Work out the finished part from the listing and answer in its coordinate system (mm). A direction names the side the tool comes from. Coordinates: 2 decimals unless noted, no trailing zeros. Write each loop counter-clockwise with the first axis right and the second up, starting at its lowest first coordinate (ties: lowest second). Pieces come first, ordered by that corner, then holes. Notation, with made-up numbers: M 75.5,80 L 87.5,80 A30 ccw 87.5,118 Z; hole C 44,7.25 d2. An arc over 180 degrees is marked long. Use CSV: the item, a comma, the result in double quotes.
Autodesk Inventor part; units mm, degrees
ref_plane "YZ Plane" through (0, 0, 0) normal (1, 0, 0) x (0, 1, 0)
ref_plane "XZ Plane" through (0, 0, 0) normal (0, 1, 0) x (-1, 0, 0)
ref_plane "XY Plane" through (0, 0, 0) normal (0, 0, 1) x (1, 0, 0)
sketch "Skizze1" plane through (0, 0, 0) normal (0, 0, 1) x (1, 0, 0)
  line L0 (-40.0777, 35.7212) -> (39.9223, 35.7212)
  line L1 (39.9223, 35.7212) -> (39.9223, -47.2788)
  line L2 (39.9223, -47.2788) -> (-40.0777, -47.2788)
  line L3 (-40.0777, -47.2788) -> (-40.0777, 35.7212)
  line L4 (-38.4777, 34.1212) -> (38.3223, 34.1212)
  line L5 (38.3223, 34.1212) -> (38.3223, -45.6788)
  line L6 (38.3223, -45.6788) -> (-38.4777, -45.6788)
  line L7 (-38.4777, -45.6788) -> (-38.4777, 34.1212)
  line L8 (-36.9777, 32.6212) -> (36.8223, 32.6212)
  line L9 (36.8223, 32.6212) -> (36.8223, -44.1788)
  line L10 (36.8223, -44.1788) -> (-36.9777, -44.1788)
  line L11 (-36.9777, -44.1788) -> (-36.9777, 32.6212)
  line L12 (-5.0777, -45.6788) -> (4.9223, -45.6788)
  line L13 (4.9223, -45.6788) -> (4.9223, -41.6788)
  line L14 (4.9223, -41.6788) -> (-5.0777, -41.6788)
  line L15 (-5.0777, -41.6788) -> (-5.0777, -45.6788)
  line L16 (-5.0777, 34.1212) -> (4.9223, 34.1212)
  line L17 (4.9223, 34.1212) -> (4.9223, 30.1212)
  line L18 (4.9223, 30.1212) -> (-5.0777, 30.1212)
  line L19 (-5.0777, 30.1212) -> (-5.0777, 34.1212)
  point P0 (0, 0)
  point P1 (-0.0777, -41.6788)
  point P2 (-0.0777, 30.1212)
  point P3 (4.9223, 32.6212)
  point P4 (-5.0777, 32.6212)
  point P5 (-5.0777, -44.1788)
  point P6 (4.9223, -44.1788)
  dimension "d0" = 80
  dimension "d1" = 83
  dimension "d2" = 1.6
  dimension "d3" = 1.5
  dimension "d4" = 1.6
  dimension "d5" = 1.5
  dimension "d6" = 1.6
  dimension "d7" = 1.5
  dimension "d8" = 1.6
  dimension "d9" = 1.5
  dimension "d10" = 10
  dimension "d11" = 4
  dimension "d12" = 40
  dimension "d13" = 4
  dimension "d14" = 10
  dimension "d16" = 40
extrude "Extrusion1" add sketch "Skizze1" along normal blind 1.5 contours L0 L1 L2 L3 | L19 L18 L17 L8 L9 L10 L13 L14 L15 L11
extrude "Extrusion2" add sketch "Skizze1" along normal blind 3 contours L4 L19 L8 L11 L10 L15 L6 L7 | L4 L5 L6 L13 L10 L9 L8 L17
extrude "Extrusion3" add sketch "Skizze1" along normal blind 8 contours L4 L17 L8 L19 | L8 L17 L18 L19 | L15 L10 L13 L6 | L15 L14 L13 L10
sketch "Skizze2" plane through (-38.4777, -45.6788, 1.5) normal (0, -1, 0) x (1, 0, 0)
  circle A0 centre (38.4, 3) radius 1
  line L0 (-1.6, 0) -> (78.4, 0)
  line L1 (33.4, 1.5) -> (33.4, 6.5)
  point P0 (38.4777, -1.5)
  dimension "d23" = 2
  dimension "d24" = 3
  dimension "d25" = 5
extrude "Extrusion4" cut sketch "Skizze2" against normal through all
properties part number "Gyrosensor_Deckel"
Item 1: A tool of negligible diameter and unlimited length cuts with its end or side. For faces 5 (the face through (0, -45.679, 3)), 6 (the face through (-1, -5, 0)), 7 (the face through (-38, 12, 3)), 8 (the face through (-0.21, 32.09, 5.49)), 9 (the face through (-5.078, 32, 5)), from which of +Z, -Z, +X, -X, +Y, -Y can it reach the whole face along a straight path? Write none if from no direction.
Answer:
face 5,"+Z, +X, -X, -Y"
face 6,"-Z, +X, -X, +Y, -Y"
face 7,"+Z, -X, +Y, -Y"
face 8,"+Y, -Y"
face 9,"+Z"
Item 2: The part is cut by section A-A (z = 4.5). Write down the section's boundary in (x, y).
Answer:
outline,"M -5.08,-45.68 L -1.08,-45.68 L -1.08,-41.68 L -5.08,-41.68 Z; M -5.08,30.12 L -1.08,30.12 L -1.08,34.12 L -5.08,34.12 Z; M 0.92,-45.68 L 4.92,-45.68 L 4.92,-41.68 L 0.92,-41.68 Z; M 0.92,30.12 L 4.92,30.12 L 4.92,34.12 L 0.92,34.12 Z"
Item 3: The part is cut by section B-B (x = 17). Write down the section's boundary in (y, z).
Answer:
outline,"M -47.28,0 L 35.72,0 L 35.72,1.5 L 34.12,1.5 L 34.12,3 L 32.62,3 L 32.62,1.5 L -44.18,1.5 L -44.18,3 L -45.68,3 L -45.68,1.5 L -47.28,1.5 Z"
Item 4: Consider probe 1 along X at (y, z) = (4, 2); probe 2 along Y at (x, z) = (2.5, 5.5); probe 3 along Y at (x, z) = (-9, 2.75). Determine where each line is inside the solid, lowest interval first.
Answer:
probe 1,"x = -38.48 to -36.98, 36.82 to 38.32"
probe 2,"y = -45.68 to -41.68, 30.12 to 34.12"
probe 3,"y = -45.68 to -44.18, 32.62 to 34.12"
Item 5: For a pull along Y with two mould halves and no side action, classify faces 1 (the face through (4.922, 32, 5)), 2 (the face through (0, 34.121, 3)), 3 (the face through (4.922, -44, 5)), 4 (the face through (38, 12, 3)) as released by +Y, released by -Y, zero draft, split by the parting line, or undercut.
Answer:
face 1,"undercut"
face 2,"released by +Y"
face 3,"undercut"
face 4,"zero draft"
Item 6: The part is cut by section C-C (y = -40). Write down the section's boundary in (x, z), then the cut area to 4 significant figures.
Answer:
outline,"M -40.08,0 L 39.92,0 L 39.92,1.5 L 38.32,1.5 L 38.32,3 L 36.82,3 L 36.82,1.5 L -36.98,1.5 L -36.98,3 L -38.48,3 L -38.48,1.5 L -40.08,1.5 Z"
area,"124.5 mm2"
Item 7: Given pin 1 (1.2 mm diameter, centred on x = 21, z = 2, fed in from +Y); pin 2 (1.5 mm diameter, centred on y = -12, z = 3, fed in from +X); pin 3 (1.2 mm diameter, centred on x = -25, z = 2.5, fed in from -Y); pin 4 (3 mm diameter, centred on x = -0.08, z = 4.5, fed in from +Y), each flat-ended and moving along its own axis, determine where each tip first touches the part or whether it passes through.
Answer:
pin 1,"stops at y = 35.72"
pin 2,"stops at x = 38.32"
pin 3,"stops at y = -45.68"
pin 4,"stops at y = 34.12"
